Answer from the drawing. Dimensions are ordinates in mm from the lowest x, y and z of the part. A direction names the side the tool comes from. Coordinates: 2 decimals unless noted, no trailing zeros. Order: outer loops, then holes, each group sorted by start corner. A loop starts at its lowest first (then second) coordinate and runs counter-clockwise, first axis right, second up. Notation, with made-up numbers: M 69,-40 L 96,-40 A14 cw 96,-27 Z; hole C 4.5,10 d1. An arc over 180 degrees is marked long. One line per question, with ' | ' between items. Start each with the question number.
1) Given P1, Ø3, axis at x = 19.5, z = 3.5, coming from the +Y side; P2, Ø0.5, axis at y = 9, z = 1, coming from the +X side; P3, Ø6, axis at x = 7, y = 6, coming from the -Z side, each flat-ended and moving along its own axis, determine where each tip first touches the part or whether it passes through.
2) Consider probe 1 along X at (y, z) = (2, 0.75); probe 2 along X at (y, z) = (12.5, 8.5); probe 3 along X at (y, z) = (10, 2.75). Determine where each line is inside the solid, lowest interval first.
3) Find section C-C, the plane y = 4. Write down the section's boundary in (x, z), plus the area to 3 significant figures.
4) Find section A-A, the plane x = 22.25. Write down the section's boundary in (y, z), plus the area to 3 significant figures.
5) A tool of negligible diameter and unlimited length cuts with its end or side. For the marked faces 1 and 2, from which of +Z, -Z, +X, -X, +Y, -Y can it reach the whole face along a straight path? Write none if from no direction.
6) Find section B-B, the plane z = 5. Write down the section's boundary in (x, y).
7) Find section D-D, the plane x = 2.5. Write down the section's boundary in (y, z), plus the area to 3 significant figures.
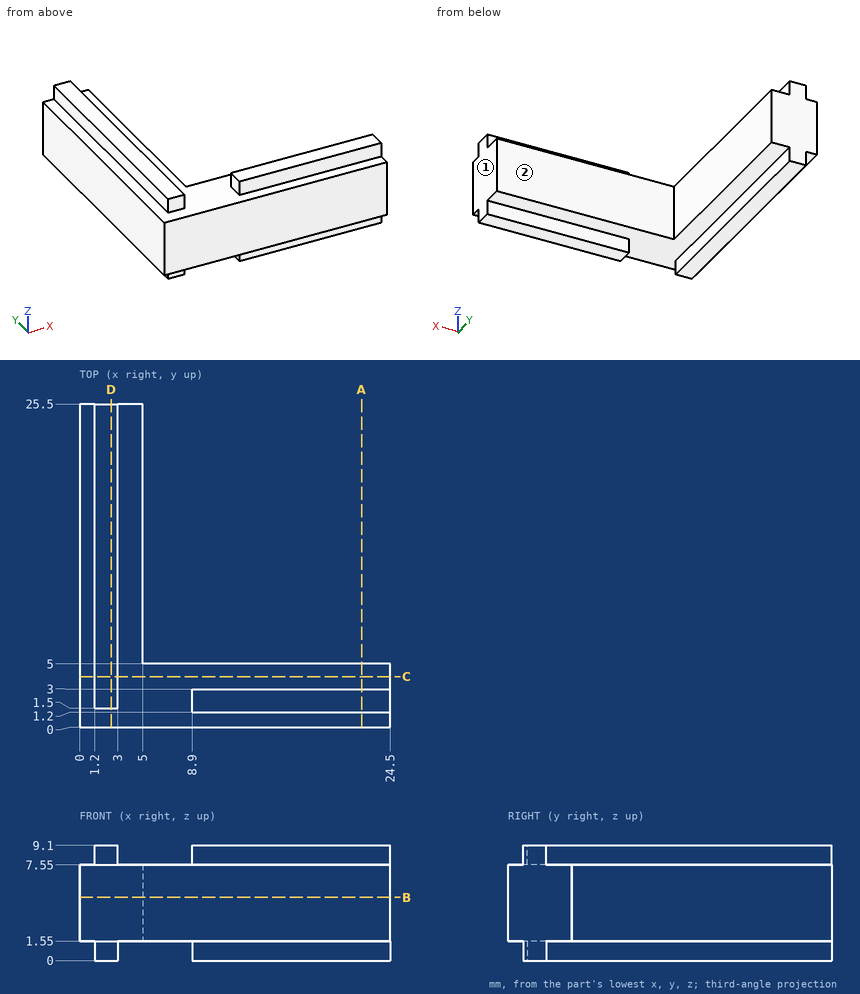
Report:
1) P1: stops at y = 5 | P2: stops at x = 3 | P3: stops at z = 1.55
2) probe 1: x = 1.2 to 3, 8.9 to 24.5 | probe 2: x = 1.2 to 3 | probe 3: x = 0 to 5
3) outline: M 0,1.55 L 1.2,1.55 L 1.2,0 L 3,0 L 3,1.55 L 24.5,1.55 L 24.5,7.55 L 3,7.55 L 3,9.1 L 1.2,9.1 L 1.2,7.55 L 0,7.55 Z | area: 153 mm^2
4) outline: M 0,1.55 L 1.2,1.55 L 1.2,0 L 3,0 L 3,1.55 L 5,1.55 L 5,7.55 L 3,7.55 L 3,9.1 L 1.2,9.1 L 1.2,7.55 L 0,7.55 Z | area: 35.6 mm^2
5) face 1: +Z, -Z, +X, +Y, -Y | face 2: +Z, -Z, +X, +Y
6) outline: M 0,0 L 24.5,0 L 24.5,5 L 5,5 L 5,25.5 L 0,25.5 Z
7) outline: M 0,1.55 L 1.5,1.55 L 1.5,0 L 25.5,0 L 25.5,9.1 L 1.5,9.1 L 1.5,7.55 L 0,7.55 Z | area: 227 mm^2
